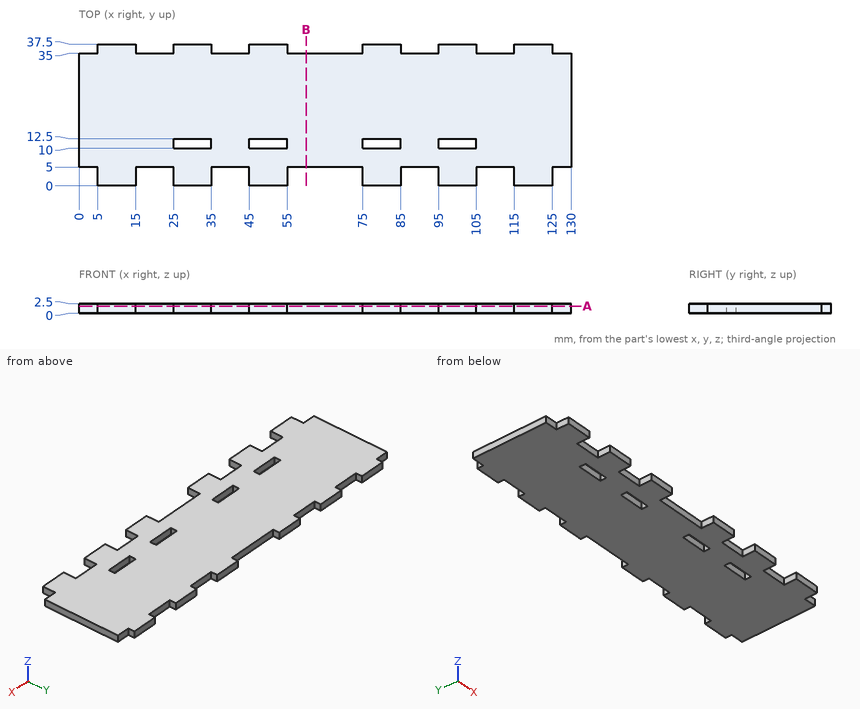
Part print with two shaded views. Sizes in mm from the minimum x, y, z corner. Coordinates: 2 decimals unless noted, no trailing zeros. Order: outer loops, then holes, each group sorted by start corner. A loop starts at its lowest first (then second) coordinate and runs counter-clockwise, first axis right, second up. Notation, with made-up numbers: (40.5, -40) - (47.5, -40) arc R24 ccw to (47.5, -26) - close; hole circle Ø7 at (-8.75, -39). An arc over 180 degrees is marked (long way). Write item = value, one per line. Start each with the question number.
1) Saw through at B-B on x = 60. Write the cut outline in (y, z), then the cut area to 3 significant figures.
2) Flat gauge pins, fed straight in: pin 1 Ø0.8 at (y, z) = (1.5, 1) entering from -X; pin 2 Ø6 at (x, y) = (28.5, 29.5) entering from -Z; pin 3 Ø0.8 at (x, z) = (64.5, 1) entering from -Y. Where does each tip first touch, or does it go through?
3) Wall check: line 1 along X through (y, z) = (2, 1); line 2 along Y through (x, z) = (25.5, 0.75); line 3 along Y through (x, z) = (91.5, 1.2). Give the ranges that are in metal, low to high. Write a range as from..to.
4) Saw through at A-A on z = 1.9. Count the separate pieces of the cut face and the enclosed holes in it, then the cut area to 3 significant figures.
From the geometry:
q1.outline = (5, 0) - (35, 0) - (35, 2.5) - (5, 2.5) - close
q1.area = 75.0 mm^2
q2.pin_1 = 5
q2.pin_2 = 0
q2.pin_3 = 5
q3.line_1 = 5..15, 25..35, 45..55, 75..85, 95..105, 115..125
q3.line_2 = 0..10, 12.5..37.5
q3.line_3 = 5..35
q4.separate_pieces = 1
q4.enclosed_holes = 4
q4.area = 4,250 mm^2
